Input: part model. Units: mm. Frame: model coordinates. A direction names the side the tool comes from. Coordinates: 2 decimals unless noted, no trailing zeros. Loops run counter-clockwise (first coordinate to the right, second up) from the corner with the lowest first, then second, coordinate; pieces in that order, holes last.
(1) Set-up query: faces 4 (the face through (58, 153, 53)), 5 (the face through (-68, 150, 70)), 6 (the face through (-68, 154, 44)). Return all of +Z, -Z, +X, -X, +Y, -Y with unobstructed straight access to the full face (end or side cutting, diameter ignored); none if empty.
(2) Section B-B, the plane y = 67. Return loops of the section in (x, z).
(3) Contact query for flat-ended pins moving along their axis: P1, Ø10, axis at x = 77.5, z = 90, coming from the -Y side; P2, Ø16, axis at x = 64.5, z = 35.5, coming from the +Y side; P3, Ø4.5, axis at x = 3.5, z = 1, coming from the +Y side. Output: stop coordinate, or through.
(4) Section D-D, the plane y = -25. Return loops of the section in (x, z).
(5) Section C-C, the plane x = -72. Return loops of the section in (y, z), then the cut area to 3 significant figures.
(6) Line query: L1, parallel to Y at x = -90.5, z = 66.5; L2, parallel to Z at x = 46.5, y = -104.5; L3, parallel to Z at x = -46.5, y = 18. Output: solid intervals per line, ascending.
(7) Section A-A, the plane z = 102. Return loops of the section in (x, y).
(8) Mould query, pull axis X, two halves, no side actions, for faces 1 (the face through (-58, 153, 53)), 2 (the face through (1, -34, -10)), 3 (the face through (-50, 1, -10)). Classes: released by +X, released by -X, zero draft, split by the parting line, or undercut.
```python
from build123d import *

# Parameters (mm, degrees)
EXTRUDE_1_DEPTH     = 4
SKETCH_2_W          = 100
SKETCH_2_H          = 72
EXTRUDE_2_DEPTH     = 20
SKETCH_4_W          = 20
SKETCH_4_H          = 4
SKETCH_7_W          = 50
SKETCH_7_H          = 10
SKETCH_9_W          = 50
SKETCH_9_H          = 10
SKETCH_12_R         = 10
CUT_EXTRUDE_1_DEPTH = 265.227174984


with BuildPart() as part:
    # 草图1 → 凸台-拉伸1 (new body)
    with BuildSketch(Plane.XY):
        Polygon((-40, 0), (40, 0), (40, -160), (78, -160), (78, 0), (78, 50), (-78, 50), (-78, 0), (-78, -160), (-40, -160), align=None)
    extrude(amount=EXTRUDE_1_DEPTH)

    # 草图2 → 凸台-拉伸2 (add)
    with BuildSketch(Plane(origin=(0, 0, 0), x_dir=(-1, 0, 0), z_dir=(0, 0, -1))):
        with Locations((0, 2)):
            Rectangle(SKETCH_2_W, SKETCH_2_H)
    extrude(amount=EXTRUDE_2_DEPTH)

    # 扫描1: sweep along a path in 草图5
    with BuildLine(Plane.ZY.offset(78)) as sweep_1_path:
        Line((0, 50), (0, 130))
        ThreePointArc((0, 130), (7.029437252, 146.970562748), (24, 154))
        Line((24, 154), (114, 154))
    # 草图4 → 扫描1 (sweep)
    with BuildSketch(Plane(origin=(0, 50, 0), x_dir=(1, 0, 0), z_dir=(0, 1, 0))):
        with Locations((-68, -2)):
            Rectangle(SKETCH_4_W, SKETCH_4_H)
        with Locations((68, -2)):
            Rectangle(SKETCH_4_W, SKETCH_4_H)
    sweep(path=sweep_1_path.line)

    # 扫描2: sweep along a path in 草图8
    with BuildLine(Plane.XY.offset(114)) as sweep_2_path:
        Line((-58, 154), (-158, 154))
    # 草图7 → 扫描2 (sweep)
    with BuildSketch(Plane(origin=(-58, 0, 0), x_dir=(0, 0, -1), z_dir=(1, 0, 0))):
        with Locations((-89, 159)):
            Rectangle(SKETCH_7_W, SKETCH_7_H)
    sweep(path=sweep_2_path.line)

    # 扫描3: sweep along a path in 草图10
    with BuildLine(Plane.XY.offset(114)) as sweep_3_path:
        Line((58, 154), (158, 154))
    # 草图9 → 扫描3 (sweep)
    with BuildSketch(Plane.ZY.offset(-58)):
        with Locations((89, 159)):
            Rectangle(SKETCH_9_W, SKETCH_9_H)
    sweep(path=sweep_3_path.line)

    # 草图12 → 切除-拉伸1 (cut, through all)
    with BuildSketch(Plane.XY.offset(114)):
        with Locations((-163, 159)):
            Circle(SKETCH_12_R)
        with Locations((163, 159)):
            Circle(SKETCH_12_R)
    extrude(amount=-CUT_EXTRUDE_1_DEPTH, mode=Mode.SUBTRACT)


solid = part.part
```
Report:
1. face 4: +Z, -Z, +Y
1. face 5: +Z, +X, -X, -Y
1. face 6: -Z, +X, -X, +Y
2. outline: (-78, 0) - (-58, 0) - (-58, 4) - (-78, 4) - close; (58, 0) - (78, 0) - (78, 4) - (58, 4) - close
3. P1: stops at y = 150
3. P2: stops at y = 154
3. P3: stops at y = 50
4. outline: (-78, 0) - (-50, 0) - (-50, -20) - (50, -20) - (50, 0) - (78, 0) - (78, 4) - (40, 4) - (40, 0) - (-40, 0) - (-40, 4) - (-78, 4) - close
5. outline: (-160, 0) - (130, 0) arc R24 ccw to (154, 24) - (154, 64) - (164, 64) - (164, 114) - (150, 114) - (150, 24) arc R20 cw to (130, 4) - (-160, 4) - close
5. area: 2,160 mm2
6. L1: y = 154 to 164
6. L2: z = 0 to 4
6. L3: z = -20 to 4
7. outline: (-154.34, 154) - (-78, 154) - (-78, 150) - (-58, 150) - (-58, 164) - (-154.34, 164) arc R10 cw to start; (58, 150) - (78, 150) - (78, 154) - (154.34, 154) arc R10 cw to (154.34, 164) - (58, 164) - close
8. face 1: undercut
8. face 2: zero draft
8. face 3: released by -X
